from build123d import *

# Parameters (mm, degrees)
BOSS_EXTRUDE1_DEPTH     = 150
CUT_EXTRUDE1_DEPTH      = 155.110350074
CUT_EXTRUDE1_DEPTH_BACK = 155.110350074
SKETCH2_R               = 2.5


with BuildPart() as part:
    # Sketch1 → Boss-Extrude1 (new body)
    with BuildSketch(Plane.XY):
        Polygon((0, 0), (25, 0), (25, -2), (-2, -2), (-2, 25), (0, 25), align=None)
    extrude(amount=BOSS_EXTRUDE1_DEPTH)

    # Sketch2 → Cut-Extrude1 (cut, two sides: drawn at the far end of the back side and taken through both)
    with BuildSketch(Plane(origin=(0, 0, 0), x_dir=(0, 0, -1), z_dir=(1, 0, 0)).offset(-CUT_EXTRUDE1_DEPTH_BACK)):
        with Locations((-120, 12.5)):
            Circle(SKETCH2_R)
        with Locations((-30, 12.5)):
            Circle(SKETCH2_R)
    extrude(amount=CUT_EXTRUDE1_DEPTH + CUT_EXTRUDE1_DEPTH_BACK, mode=Mode.SUBTRACT)


solid = part.part
For this review, take the finished solid that the model builds, in its own axes (mm). A direction names the side the tool comes from. Round coordinates to 2 decimals unless told otherwise and drop trailing zeros. Order: outer loops, then holes, each group sorted by start corner. A loop starts at its lowest first (then second) coordinate and runs counter-clockwise, first axis right, second up. Notation, with made-up numbers: M -26.5,-8.5 L 25.5,-8.5 A37 cw 25.5,30.5 Z; hole C -18,38 d1. An arc over 180 degrees is marked long. Use a Markdown table: item, result. Add a question column.
Item 1: To check wall thickness, follow line 1 along Z through (x, y) = (-0.75, 12.5); line 2 along Y through (x, z) = (-0.7, 30); line 3 along X through (y, z) = (21.75, 127). State the ranges of each line that lie inside material, in increasing order.
Item 2: Add section B-B, the plane z = 120. Give the boundary of the cut face in (x, y), then the cut area to 3 significant figures.
Item 3: Add section C-C, the plane z = 72.5. Give the boundary of the cut face in (x, y), then the cut area to 3 significant figures.
Item 4: Tool access review of faces 1 (the flat face through (5.6, -0.4, 0)), 2 (the flat face through (0, 13, 74)): name each direction out of +Z, -Z, +X, -X, +Y, -Y from which nothing blocks a thin tool from reaching the whole face with its end or side.
Item 5: Insertion check: pin 1 (2 mm diameter, centred on x = 9, z = 28, fed in from +Y); pin 2 (3 mm diameter, centred on y = 12.5, z = 120, fed in from +X). Each pin has a flat end and moves straight along its axis. Give the tip position at first contact, or say it passes through.
Item 6: Add section D-D, the plane x = 20.25. Give the boundary of the cut face in (y, z), then the cut area to 3 significant figures.
Item 7: Mouldability with a two-part tool opening along Y and no side actions: class faces 3 (the cylindrical face through (-1.014, 13.251, 117.615)), 4 (the flat face through (12, 0, 74)), 5 (the flat face through (-2, 11, 74)) as released by +Y, released by -Y, zero draft, split by the parting line, or undercut.
Item 8: Add section A-A, the plane y = 12.5. Give the boundary of the cut face in (x, z), then the cut area to 3 significant figures.
Geometry results:
| question | item | result |
|---|---|---|
| 1 | line 1 | z = 0 to 27.5, 32.5 to 117.5, 122.5 to 150 |
| 1 | line 2 | y = -2 to 10, 15 to 25 |
| 1 | line 3 | x = -2 to 0 |
| 2 | outline | M -2,-2 L 25,-2 L 25,0 L 0,0 L 0,10 L -2,10 Z; M -2,15 L 0,15 L 0,25 L -2,25 Z |
| 2 | area | 94.0 mm² |
| 3 | outline | M -2,-2 L 25,-2 L 25,0 L 0,0 L 0,25 L -2,25 Z |
| 3 | area | 104 mm² |
| 4 | face 1 | -Z, +X, -X, +Y, -Y |
| 4 | face 2 | +Z, -Z, +X, +Y |
| 5 | pin 1 | stops at y = 0 |
| 5 | pin 2 | passes through |
| 6 | outline | M -2,0 L 0,0 L 0,150 L -2,150 Z |
| 6 | area | 300 mm² |
| 7 | face 3 | undercut |
| 7 | face 4 | released by +Y |
| 7 | face 5 | zero draft |
| 8 | outline | M -2,0 L 0,0 L 0,27.5 L -2,27.5 Z; M -2,32.5 L 0,32.5 L 0,117.5 L -2,117.5 Z; M -2,122.5 L 0,122.5 L 0,150 L -2,150 Z |
| 8 | area | 280 mm² |
